Could you check a few things on this model? Use its own coordinates, in mm. A direction names the side the tool comes from. Coordinates: 2 decimals unless noted, no trailing zeros. Loops run counter-clockwise (first coordinate to the right, second up) from the corner with the lowest first, then second, coordinate; pieces in that order, holes last.
1) If I drill on line 1 along Y through (x, z) = (0, -18) (3 decimals); line 2 along Y through (x, z) = (0, -18.95) (3 decimals); line 3 along Y through (x, z) = (3, -21) (3 decimals), over which ranges is the centre line in solid material (lowest first)?
2) Thinking about a two-plate mould opening in X: for faces 1 (the face through (134.268, 130.796, -93.916)), 2 (the face through (-58, 28, -19.05)), 3 (the face through (-2, -136.525, -94)), 4 (the face through (-133.971, 131.093, -93.916)), which applies, released by +X, released by -X, zero draft, split by the parting line, or undercut?
3) Imagine slicing it at D-D on x = -110. Please give me the cut outline in (y, z) (3 decimals).
4) For faces 5 (the face through (120.65, -24, -104)), 6 (the face through (2, 136.525, -94)), 7 (the face through (-2, 111.125, -9)), which set-ups out of +Z, -Z, +X, -X, +Y, -Y let a thin tool reach every point of the face, with its end or its side?
5) Will these pins go through, and if not, where does the flat tip stop? P1, Ø10, axis at x = -62, y = 19.5, coming from the +Z side; P2, Ø5, axis at x = -123.5, z = -112, coming from the +Y side; P3, Ø6, axis at x = 91, y = 19, coming from the -Z side.
6) Imagine slicing it at C-C on z = -135. Please give me the cut outline in (x, y) (3 decimals).
7) Imagine slicing it at B-B on x = 0. Give the number of separate pieces and of enclosed holes in the cut face, plus the area to 3 significant figures.
```python
from build123d import *

# Parameters (mm, degrees)
F1_DEPTH = 190.5
F2_W     = 50.8
F2_H     = 19.05
F3_DEPTH = 6.35
F4_W     = 50.8
F4_H     = 19.05
F5_DEPTH = 6.35
F0_W     = 241.3
F0_H     = 184.15
F0_R     = 71
F0_H_2   = 38.1
F6_DEPTH = 19.05
F7_R     = 19.04999


# Not quite as in the source:
# - a fillet or chamfer is up to 0.001 mm smaller than in the source, because OpenCascade refuses the exact size


with BuildPart() as f1:
    # F0 (on Top) → F1 (new body)
    with BuildSketch(Plane.XY):
        with BuildLine():
            Line((-120.65, -136.525), (120.65, -136.525))
            ThreePointArc((120.65, -136.525), (134.1203841816, -130.9453841816), (139.7, -117.475))
            Line((139.7, -117.475), (139.7, 117.475))
            Line((139.7, 117.475), (127, 117.475))
            Line((127, 117.475), (127, 66.675))
            Line((127, 66.675), (120.65, 66.675))
            Line((120.65, 66.675), (120.65, -117.475))
            Line((120.65, -117.475), (-120.65, -117.475))
            Line((-120.65, -117.475), (-120.65, 66.675))
            Line((-120.65, 66.675), (-127, 66.675))
            Line((-127, 66.675), (-127, 117.475))
            Line((-127, 117.475), (-139.7, 117.475))
            Line((-139.7, 117.475), (-139.7, -117.475))
            ThreePointArc((-139.7, -117.475), (-134.1203841816, -130.9453841816), (-120.65, -136.525))
        make_face()
        with BuildLine():
            Line((127, 117.475), (139.7, 117.475))
            ThreePointArc((139.7, 117.475), (134.1203841816, 130.9453841816), (120.65, 136.525))
            Line((120.65, 136.525), (-120.65, 136.525))
            ThreePointArc((-120.65, 136.525), (-134.1203841816, 130.9453841816), (-139.7, 117.475))
            Line((-139.7, 117.475), (-127, 117.475))
            Line((-127, 117.475), (127, 117.475))
        make_face()
    extrude(amount=-F1_DEPTH)

    # F2 (on face) → F3 (join)
    with BuildSketch(Plane(origin=(127, 0, 0), x_dir=(0, -1, 0), z_dir=(-1, 0, 0))):
        with Locations((-92.075, -9.525)):
            Rectangle(F2_W, F2_H)
    extrude(amount=F3_DEPTH)

    # F4 (on face) → F5 (join)
    with BuildSketch(Plane.YZ.offset(-127)):
        with Locations((92.075, -9.525)):
            Rectangle(F4_W, F4_H)
    extrude(amount=F5_DEPTH)

    # F0 (on Top) → F6 (join)
    with BuildSketch(Plane.XY):
        with Locations((0, -25.4)):
            Rectangle(F0_W, F0_H)
        with Locations((0, -31.75)):
            Circle(F0_R, mode=Mode.SUBTRACT)
        Polygon((127, 66.675), (127, 117.475), (-127, 117.475), (-127, 66.675), (-120.65, 66.675), (120.65, 66.675), align=None)
        with Locations((0, 92.075)):
            Rectangle(F0_W, F0_H_2, mode=Mode.SUBTRACT)
    extrude(amount=-F6_DEPTH)

    # F7 (radius 19.05 in the source; OpenCascade refuses exactly that, so slightly less here)
    f7_edges = [f1.edges().sort_by_distance(p)[0] for p in [
        (-71, -31.75, 0),
    ]]
    fillet(f7_edges, radius=F7_R)


solid = f1.part
```
Filled in:
1. line 1: y = -136.525 to -102.779, 39.279 to 73.025, 111.125 to 136.525
1. line 2: y = -136.525 to -102.75, 39.25 to 73.025, 111.125 to 136.525
1. line 3: y = -136.525 to -117.475, 117.475 to 136.525
2. face 1: released by +X
2. face 2: undercut
2. face 3: zero draft
2. face 4: released by -X
3. outline: (-136.525, -190.5) - (-117.475, -190.5) - (-117.475, -19.05) - (73.025, -19.05) - (73.025, 0) - (-136.525, 0) - close; (111.125, -19.05) - (117.475, -19.05) - (117.475, -190.5) - (136.525, -190.5) - (136.525, 0) - (111.125, 0) - close
4. face 5: -Z
4. face 6: +Z, -Z, +X, -X, +Y
4. face 7: +Z, -Z
5. P1: stops at z = -0.57
5. P2: stops at y = 136.52
5. P3: stops at z = -19.05
6. outline: (-139.7, -117.475) arc R19.05 ccw to (-120.65, -136.525) - (120.65, -136.525) arc R19.05 ccw to (139.7, -117.475) - (139.7, 117.475) arc R19.05 ccw to (120.65, 136.525) - (-120.65, 136.525) arc R19.05 ccw to (-139.7, 117.475) - close; hole (-127, 66.675) - (-120.65, 66.675) - (-120.65, -117.475) - (120.65, -117.475) - (120.65, 66.675) - (127, 66.675) - (127, 117.475) - (-127, 117.475) - close
7. separate pieces: 3
7. enclosed holes: 0
7. area: 8,150 mm2
